from build123d import *

# Parameters (mm, degrees)
ESBO_O1_R                = 110
RESSALTO_EXTRUS_O1_DEPTH = 1550
RESSALTO_EXTRUS_O2_REACH = 287
ESBO_O3_R                = 25


with BuildPart() as part:
    # Esboço1 → Ressalto-extrusão1 (new body)
    with BuildSketch(Plane.XY):
        Circle(ESBO_O1_R)
    extrude(amount=RESSALTO_EXTRUS_O1_DEPTH)

    # Esboço3 → Ressalto-extrusão2 (add, up to next)
    with BuildSketch(Plane(origin=(0, 175, 0), x_dir=(1, 0, 0), z_dir=(0, 1, 0)), mode=Mode.PRIVATE) as ressalto_extrus_o2_sk1:
        with Locations((0, -600)):
            Circle(ESBO_O3_R)
    ressalto_extrus_o2_tool1 = extrude(ressalto_extrus_o2_sk1.sketch, amount=-RESSALTO_EXTRUS_O2_REACH, mode=Mode.PRIVATE) - part.part
    add(ressalto_extrus_o2_tool1.solids().sort_by_distance((0, 175, 600))[0])
    # Esboço3 → Ressalto-extrusão2 (add, up to next)
    with BuildSketch(Plane(origin=(0, 175, 0), x_dir=(1, 0, 0), z_dir=(0, 1, 0)), mode=Mode.PRIVATE) as ressalto_extrus_o2_sk2:
        with Locations((0, -950)):
            Circle(ESBO_O3_R)
    ressalto_extrus_o2_tool2 = extrude(ressalto_extrus_o2_sk2.sketch, amount=-RESSALTO_EXTRUS_O2_REACH, mode=Mode.PRIVATE) - part.part
    add(ressalto_extrus_o2_tool2.solids().sort_by_distance((0, 175, 950))[0])


solid = part.part
Verification items for the finished model (mm, model axes). A direction names the side the tool comes from. Give positions to 0.01 mm unless a question says otherwise; leave off trailing zeros. Write each loop counter-clockwise with the first axis right and the second up, starting at its lowest first coordinate (ties: lowest second). Pieces come first, ordered by that corner, then holes. Notation, with made-up numbers: (36, 33) -> (44, 33) arc R9 cw to (44, 42) -> close; hole circle Ø8 at (54, 81). An arc over 180 degrees is marked (long way). Use CSV: the item, a comma, the result in double quotes.
(1) Sectioned sample at A-A (x = 0). Record the cut outline in (y, z), plus the area to 4 significant figures.
Derived:
outline,"(-110, 0) -> (110, 0) -> (110, 575) -> (175, 575) -> (175, 625) -> (110, 625) -> (110, 925) -> (175, 925) -> (175, 975) -> (110, 975) -> (110, 1550) -> (-110, 1550) -> close"
area,"347,500 mm^2"
(2) Sectioned sample at B-B (z = 1289.5). Record the cut outline in (x, y).
Derived:
outline,"circle Ø220 at (0, 0)"
(3) Sectioned sample at C-C (y = -67). Record the cut outline in (x, z).
Derived:
outline,"(-87.24, 0) -> (87.24, 0) -> (87.24, 1550) -> (-87.24, 1550) -> close"
(4) Material ranges on L1, parallel to Z at x = 3.5, y = 163.5; L2, parallel to Y at x = 8.5, z = 1284; L3, parallel to X at y = 67, z = 463, recorded low to high.
Derived:
L1,"z = 575.25 to 624.75, 925.25 to 974.75"
L2,"y = -109.67 to 109.67"
L3,"x = -87.24 to 87.24"
(5) Set-up check for faces 4 (the flat face through (-2, 2, 1550)), 5 (the cylindrical face through (11.5, 141.5, 972.2)): record each of +Z, -Z, +X, -X, +Y, -Y from which the full face is reachable in a straight line by a thin tool's end or side.
Derived:
face 4,"+Z, +X, -X, +Y, -Y"
face 5,"+Y"
(6) Go/stop test with flat-tipped pins: pin 1 (3 mm diameter, centred on y = -19, z = 1314, fed in from -X); pin 2 (12 mm diameter, centred on y = 37.5, z = 1391.5, fed in from +X); pin 3 (10 mm diameter, centred on y = -51, z = 179.5, fed in from +X). Record where each tip stops, or that it passes through.
Derived:
pin 1,"stops at x = -108.6"
pin 2,"stops at x = 105.39"
pin 3,"stops at x = 99.92"
(7) Release check for a two-part mould opening along Z. For faces 1 (the cylindrical face through (11.5, 141.5, 622.2)), 2 (the flat face through (0, 175, 950)), 3 (the flat face through (-2, 2, 0)) record: +Z half, -Z half, draft (parallel to the pull), parting line (faces both ways), or undercut.
Derived:
face 1,"undercut"
face 2,"draft"
face 3,"-Z half"
(8) Sectioned sample at D-D (z = 950). Record the cut outline in (x, y), plus the area to 3 significant figures.
Derived:
outline,"(-25, 107.12) arc R110 ccw (long way) to (25, 107.12) -> (25, 175) -> (-25, 175) -> close"
area,"41,300 mm^2"
